The listing builds one solid part. Answer for the finished solid, in the listing's coordinates (mm). A direction names the side the tool comes from. Give positions to 0.01 mm unless a question says otherwise; leave off trailing zeros. Write each loop counter-clockwise with the first axis right and the second up, starting at its lowest first coordinate (ties: lowest second). Pieces come first, ordered by that corner, then holes. Notation, with made-up numbers: M 52.5,9 L 110.5,9 A26 cw 110.5,41 Z; hole C -11,17 d3. An arc over 180 degrees is marked long. Answer as a JSON object with one key per item and string values.
```python
from build123d import *

# Parameters (mm, degrees)
SKETCH1_R           = 11
SKETCH1_R_2         = 1.25
BOSS_EXTRUDE2_DEPTH = 2.5
SKETCH2_R           = 5
BOSS_EXTRUDE3_DEPTH = 18
SKETCH3_R           = 5
SKETCH3_R_2         = 2
BOSS_EXTRUDE4_DEPTH = 2


with BuildPart() as part:
    # Sketch1 → Boss-Extrude2 (new body)
    with BuildSketch(Plane(origin=(0, 0, 0), x_dir=(1, 0, 0), z_dir=(0, 1, 0))):
        with Locations(Location((0, 0, 0), (0, 0, 270))):
            Circle(SKETCH1_R)
        with Locations(Location((-7.8, 0, 0), (0, 0, 270))):
            Circle(SKETCH1_R_2, mode=Mode.SUBTRACT)
        with Locations(Location((0, 7.8, 0), (0, 0, 270))):
            Circle(SKETCH1_R_2, mode=Mode.SUBTRACT)
        with Locations(Location((7.8, 0, 0), (0, 0, 270))):
            Circle(SKETCH1_R_2, mode=Mode.SUBTRACT)
        with Locations(Location((0, -7.8, 0), (0, 0, 270))):
            Circle(SKETCH1_R_2, mode=Mode.SUBTRACT)
    extrude(amount=BOSS_EXTRUDE2_DEPTH)

    # Sketch2 → Boss-Extrude3 (add)
    with BuildSketch(Plane(origin=(0, 2.5, 0), x_dir=(1, 0, 0), z_dir=(0, 1, 0))):
        with Locations(Location((0, 0, 0), (0, 0, 270))):
            Circle(SKETCH2_R)
    extrude(amount=BOSS_EXTRUDE3_DEPTH)

    # Sketch3 → Boss-Extrude4 (add)
    with BuildSketch(Plane(origin=(0, 20.5, 0), x_dir=(1, 0, 0), z_dir=(0, 1, 0))):
        with Locations(Location((0, 0, 0), (0, 0, 270))):
            Circle(SKETCH3_R)
        with Locations(Location((0, 0, 0), (0, 0, 270))):
            Circle(SKETCH3_R_2, mode=Mode.SUBTRACT)
    extrude(amount=BOSS_EXTRUDE4_DEPTH)


solid = part.part
```
1. A cutting plane is placed at A-A, the plane z = 0. Give the vertices of the cut face in (x, y), plus the area to 4 significant figures.
Verdict:
{"outline": "M -11,0 L -9.05,0 L -9.05,2.5 L -11,2.5 Z; M -6.55,0 L 6.55,0 L 6.55,2.5 L 5,2.5 L 5,22.5 L 2,22.5 L 2,20.5 L -2,20.5 L -2,22.5 L -5,22.5 L -5,2.5 L -6.55,2.5 Z; M 9.05,0 L 11,0 L 11,2.5 L 9.05,2.5 Z", "area": "234.5 mm2"}
2. Flat-ended cylindrical pins translate along their axes: pin 1 (10 mm diameter, centred on y = 9, z = 7.5, fed in from +X); pin 2 (6 mm diameter, centred on x = -7, y = 12.5, fed in from -Z); pin 3 (10 mm diameter, centred on x = -5.5, y = 13.5, fed in from -Z). Find the tip coordinate at first contact, or state that the pin passes through.
Verdict:
{"pin 1": "stops at x = 4.33", "pin 2": "stops at z = -3", "pin 3": "stops at z = -4.97"}
3. A cutting plane is placed at D-D, the plane z = -7.5. Give the vertices of the cut face in (x, y), plus the area to 3 significant figures.
Verdict:
{"outline": "M -8.05,0 L -1.21,0 L -1.21,2.5 L -8.05,2.5 Z; M 1.21,0 L 8.05,0 L 8.05,2.5 L 1.21,2.5 Z", "area": "34.2 mm2"}
4. A cutting plane is placed at C-C, the plane x = 8.25. Give the vertices of the cut face in (y, z).
Verdict:
{"outline": "M 0,-7.28 L 2.5,-7.28 L 2.5,-1.17 L 0,-1.17 Z; M 0,1.17 L 2.5,1.17 L 2.5,7.28 L 0,7.28 Z"}
5. For faces 1 (the cylindrical face through (0.38, 1.23, -6.61)), 2 (the flat face through (0, 20.5, 0)), determine the directions among +Z, -Z, +X, -X, +Y, -Y from which every point of the face is accessible in a straight line to the end or side of a thin tool.
Verdict:
{"face 1": "+Y, -Y", "face 2": "+Y"}
6. Consider line 1 along X through (y, z) = (0.6, 0); line 2 along Y through (x, z) = (-5.5, 9.25); line 3 along X through (y, z) = (1.85, 7.8). Determine where each line is inside the solid, lowest interval first.
Verdict:
{"line 1": "x = -11 to -9.05, -6.55 to 6.55, 9.05 to 11", "line 2": "y = 0 to 2.5", "line 3": "x = -7.76 to -1.25, 1.25 to 7.76"}
7. A cutting plane is placed at B-B, the plane x = 0. Give the vertices of the cut face in (y, z).
Verdict:
{"outline": "M 0,-11 L 2.5,-11 L 2.5,-9.05 L 0,-9.05 Z; M 0,-6.55 L 2.5,-6.55 L 2.5,-5 L 22.5,-5 L 22.5,-2 L 20.5,-2 L 20.5,2 L 22.5,2 L 22.5,5 L 2.5,5 L 2.5,6.55 L 0,6.55 Z; M 0,9.05 L 2.5,9.05 L 2.5,11 L 0,11 Z"}
8. The mould has two halves that part along Z. Classify faces 3 (the cylindrical face through (-2, 21, 0)), 4 (the cylindrical face through (0.05, 1.23, 6.55)), 5 (the flat face through (-5, 2.5, 2)), 6 (the cylindrical face through (-10.74, 1.23, -2.38)): released by +Z, released by -Z, zero draft, split by the parting line, or undercut.
Verdict:
{"face 3": "undercut", "face 4": "undercut", "face 5": "zero draft", "face 6": "split by the parting line"}
